```python
from build123d import *

# Parameters (mm, degrees)
BOSS_EXTRUDE1_DEPTH = 5.715


with BuildPart() as part:
    # Model → Boss-Extrude1 (new body)
    with BuildSketch(Plane.XY):
        Polygon((803.25976, 23.2006394), (810.71212, 23.2006394), (810.71212, 28.91536), (822.14212, 28.91536), (822.14212, 23.2006394), (833.57212, 23.2006394), (833.57212, 28.91536), (845.00212, 28.91536), (845.00212, 23.2006394), (852.4494, 23.2006394), (852.4494, 279.63114), (845.00212, 279.63114), (845.00212, 273.91614), (833.57212, 273.91614), (833.57212, 279.63114), (822.14212, 279.63114), (822.14212, 273.91614), (810.71212, 273.91614), (810.71212, 279.63114), (803.25976, 279.63114), (803.25976, 251.055124), (803.25976, 250.316746), (803.65346, 248.098056), (804.54246, 245.775988), (804.79138, 245.340378), (805.04538, 244.906546), (806.60748, 242.974368), (808.54296, 241.407696), (808.97476, 241.156744), (809.4091, 240.906046), (811.34204, 239.34039), (812.90922, 237.408466), (813.16068, 236.972856), (813.4096, 236.539024), (814.30368, 234.216956), (814.69484, 231.998266), (814.69484, 231.25811), (814.69484, 71.572628), (814.68976, 71.070978), (814.30368, 68.615306), (813.4096, 66.293238), (813.16068, 65.857882), (812.90922, 65.423796), (811.34204, 63.491872), (809.4091, 61.924946), (808.97476, 61.673994), (808.54296, 61.423296), (806.60748, 59.857894), (805.04538, 57.925716), (804.79138, 57.49036), (804.54246, 57.056274), (803.65346, 54.734206), (803.25976, 52.515516), (803.25976, 51.775868), align=None)
        Polygon((820.40984, 254.28448), (820.40984, 259.99948), (826.12484, 259.99948), (826.12484, 248.570496), (820.40984, 248.570496), align=None, mode=Mode.SUBTRACT)
        Polygon((820.40984, 231.424988), (820.40984, 237.141004), (826.12484, 237.141004), (826.12484, 225.710496), (820.40984, 225.710496), align=None, mode=Mode.SUBTRACT)
        Polygon((820.40984, 208.566004), (820.40984, 214.28075), (826.12484, 214.28075), (826.12484, 202.849988), (820.40984, 202.849988), align=None, mode=Mode.SUBTRACT)
        Polygon((820.40984, 185.70575), (820.40984, 191.420496), (826.12484, 191.420496), (826.12484, 179.991004), (820.40984, 179.991004), align=None, mode=Mode.SUBTRACT)
        Polygon((820.40984, 162.845496), (820.40984, 168.560496), (826.12484, 168.560496), (826.12484, 157.13075), (820.40984, 157.13075), align=None, mode=Mode.SUBTRACT)
        Polygon((820.40984, 139.985496), (820.40984, 145.699988), (826.12484, 145.699988), (826.12484, 134.270496), (820.40984, 134.270496), align=None, mode=Mode.SUBTRACT)
        Polygon((820.40984, 117.124988), (820.40984, 122.841004), (826.12484, 122.841004), (826.12484, 111.410496), (820.40984, 111.410496), align=None, mode=Mode.SUBTRACT)
        Polygon((820.40984, 94.266004), (820.40984, 99.98075), (826.12484, 99.98075), (826.12484, 88.549988), (820.40984, 88.549988), align=None, mode=Mode.SUBTRACT)
        Polygon((820.40984, 71.40575), (820.40984, 77.120496), (826.12484, 77.120496), (826.12484, 65.691004), (820.40984, 65.691004), align=None, mode=Mode.SUBTRACT)
        Polygon((820.40984, 48.545496), (820.40984, 54.260496), (826.12484, 54.260496), (826.12484, 42.83075), (820.40984, 42.83075), align=None, mode=Mode.SUBTRACT)
    extrude(amount=BOSS_EXTRUDE1_DEPTH)


solid = part.part
```
Geometry: final body of the model. Coordinates: model frame, mm. A direction names the side the tool comes from. Give positions to 0.01 mm unless a question says otherwise; leave off trailing zeros. Order: outer loops, then holes, each group sorted by start corner. A loop starts at its lowest first (then second) coordinate and runs counter-clockwise, first axis right, second up. Notation, with made-up numbers: M 30.5,-29.75 L 62.5,-29.75 A34 ccw 62.5,6.25 Z; hole C 66,-36.75 d2. An arc over 180 degrees is marked long. Answer as CSV lines item,"result". Start each with the question number.
1) Mould query, pull axis Y, two halves, no side actions, for faces 6 (the flat face through (810.712, 277, 3)), 7 (the flat face through (828, 23.201, 3)), 8 (the flat face through (820.41, 163, 3)). Classes: +Y half, -Y half, draft (parallel to the pull), parting line (faces both ways), or undercut.
2) Cut plane A-A (y = 138). Output: boundary loops of the cut face in (x, z) (3 decimals), then the cut area to 3 significant figures.
3) Line query: line 1 (X direction, y = 96, z = 4.3); line 2 (X direction, y = 44.5, z = 2.25); line 3 (X direction, y = 220, z = 4.85). Output: solid intervals per line, ascending. Write a range as from..to.
4) Cut plane B-B (y = 47). Output: boundary loops of the cut face in (x, z) (3 decimals).
5) Set-up query: faces 1 (the flat face through (822.142, 26, 3)), 2 (the flat face through (807, 23.201, 3)), 3 (the flat face through (845.002, 277, 3)), 4 (the flat face through (814.695, 153, 3)), 5 (the flat face through (820.41, 231, 3)). Return all of +Z, -Z, +X, -X, +Y, -Y with unobstructed straight access to the full face (end or side cutting, diameter ignored); none if empty.
6) First-contact query: P1, Ø3, axis at y = 187, z = 3.5, coming from the -X side; P2, Ø10, axis at x = 809, y = 129, coming from the +Z side. Flat tips, straight axial feed; report the tip coordinate or a pass-through.
7) Cut plane C-C (z = 3.05). State how many separate pieces and enclosed holes the cut face has, then the cut area to 3 significant figures.
8) Cut plane D-D (x = 817). Output: boundary loops of the cut face in (y, z) (3 decimals), then the cut area to 3 significant figures.
Findings below:
1,face 6,"draft"
1,face 7,"-Y half"
1,face 8,"undercut"
2,outline,"M 814.695,0 L 820.41,0 L 820.41,5.715 L 814.695,5.715 Z; M 826.125,0 L 852.449,0 L 852.449,5.715 L 826.125,5.715 Z"
2,area,"183 mm²"
3,line 1,"x = 814.69..820.41, 826.12..852.45"
3,line 2,"x = 803.26..820.41, 826.12..852.45"
3,line 3,"x = 814.69..852.45"
4,outline,"M 803.26,0 L 820.41,0 L 820.41,5.715 L 803.26,5.715 Z; M 826.125,0 L 852.449,0 L 852.449,5.715 L 826.125,5.715 Z"
5,face 1,"+Z, -Z, -Y"
5,face 2,"+Z, -Z, +X, -X, -Y"
5,face 3,"+Z, -Z, +Y"
5,face 4,"+Z, -Z, -X"
5,face 5,"+Z, -Z"
6,P1,"stops at x = 814.69"
6,P2,"passes through"
7,separate pieces,"1"
7,enclosed holes,"10"
7,area,"9,650 mm²"
8,outline,"M 28.915,0 L 273.916,0 L 273.916,5.715 L 28.915,5.715 Z"
8,area,"1,400 mm²"
